from build123d import *
from OCP.BRepFilletAPI import BRepFilletAPI_MakeChamfer

# Parameters (mm, degrees)
SZKIC1_W                        = 58
SZKIC1_H                        = 20
DODANIE_WYCI_GNI_CIE1_DEPTH     = 5
SZKIC2_W                        = 15
SZKIC2_H                        = 5
DODANIE_WYCI_GNI_CIE2_DEPTH     = 58
DODANIE_WYCI_GNI_CIE3_DEPTH     = 20
DODANIE_WYCI_GNI_CIE4_DEPTH     = 10
WYTNIJ_WYCI_GNI_CIE2_DEPTH      = 50.950375374
WYTNIJ_WYCI_GNI_CIE2_DEPTH_BACK = 50.950375374
SZKIC6_W                        = 58
SZKIC6_H                        = 5
DODANIE_WYCI_GNI_CIE5_DEPTH     = 20
SZKIC7_R                        = 2
WYTNIJ_WYCI_GNI_CIE3_DEPTH      = 10
DODANIE_WYCI_GNI_CIE8_DEPTH     = 10
SZKIC11_W                       = 10.2
SZKIC11_H                       = 10.2
DODANIE_WYCI_GNI_CIE9_DEPTH     = 5
SFAZOWANIE2_SIZE                = 5
SZKIC12_W                       = 10
SZKIC12_H                       = 20
WYTNIJ_WYCI_GNI_CIE4_DEPTH      = 10
SZKIC13_R                       = 1.7
WYTNIJ_WYCI_GNI_CIE5_DEPTH      = 60.991999467
DODANIE_WYCI_GNI_CIE11_DEPTH    = 5
SFAZOWANIE6_SIZE                = 5
SFAZOWANIE6_SIZE2               = 8.660254038


with BuildPart() as part:
    # Szkic1 → Dodanie-wyciągnięcie1 (new body)
    with BuildSketch(Plane.XY):
        Rectangle(SZKIC1_W, SZKIC1_H)
    extrude(amount=DODANIE_WYCI_GNI_CIE1_DEPTH)

    # Szkic2 → Dodanie-wyciągnięcie2 (add)
    with BuildSketch(Plane(origin=(29, 0, 0), x_dir=(0, 0, -1), z_dir=(1, 0, 0))):
        with Locations((-2.5, 12.5)):
            Rectangle(SZKIC2_W, SZKIC2_H)
    extrude(amount=-DODANIE_WYCI_GNI_CIE2_DEPTH)

    # Szkic3 → Dodanie-wyciągnięcie3 (add)
    with BuildSketch(Plane.XZ.offset(10)):
        Polygon((-34, 5), (-29, 0), (-29, 5), (-24, 5), (-29, 10), (-34, 10), align=None)
    extrude(amount=-DODANIE_WYCI_GNI_CIE3_DEPTH)

    # Szkic5 → Dodanie-wyciągnięcie4 (add)
    with BuildSketch(Plane.XY.offset(5)):
        Polygon((14.2, 20.2), (14.2, 10), (19, 10), (19, 35.2), (-16, 35.2), (-16, 10), (4, 10), (4, 20.2), align=None)
    extrude(amount=-DODANIE_WYCI_GNI_CIE4_DEPTH)

    # Szkic5<3> → Wytnij-wyciągnięcie2 (cut, two sides: drawn at the far end of the back side and taken through both)
    with BuildSketch(Plane.XY.offset(5).offset(-WYTNIJ_WYCI_GNI_CIE2_DEPTH_BACK)):
        Polygon((4, 10), (14.2, 10), (14.2, 15), (14.2, 20.2), (4, 20.2), (4, 15), align=None)
    extrude(amount=WYTNIJ_WYCI_GNI_CIE2_DEPTH + WYTNIJ_WYCI_GNI_CIE2_DEPTH_BACK, mode=Mode.SUBTRACT)

    # Szkic6 → Dodanie-wyciągnięcie5 (add)
    with BuildSketch(Plane(origin=(0, 10, 0), x_dir=(1, 0, 0), z_dir=(0, 1, 0))):
        with Locations((0, -7.5)):
            Rectangle(SZKIC6_W, SZKIC6_H)
    extrude(amount=-DODANIE_WYCI_GNI_CIE5_DEPTH)

    # Szkic7 → Wytnij-wyciągnięcie3 (cut)
    with BuildSketch(Plane.XZ.offset(10)):
        with Locations(Location((-19, 5, 0), (0, 0, 270))):
            Circle(SZKIC7_R)
        with Locations(Location((11, 5, 0), (0, 0, 270))):
            Circle(SZKIC7_R)
    extrude(amount=-WYTNIJ_WYCI_GNI_CIE3_DEPTH, mode=Mode.SUBTRACT)

    # Szkic10 → Dodanie-wyciągnięcie8 (add)
    with BuildSketch(Plane(origin=(0, 0, -5), x_dir=(-1, 0, 0), z_dir=(0, 0, -1))):
        Polygon((16, 10), (16, 15), (16, 35.2), (-19, 35.2), (-19, 15), (-29, 15), (-29, 10), (-14.2, 10), (-14.2, 20.2), (-4, 20.2), (-4, 10), align=None)
    extrude(amount=DODANIE_WYCI_GNI_CIE8_DEPTH)

    # Szkic11 → Dodanie-wyciągnięcie9 (add)
    with BuildSketch(Plane(origin=(0, 0, -15), x_dir=(-1, 0, 0), z_dir=(0, 0, -1))):
        with Locations((-9.1, 15.1)):
            Rectangle(SZKIC11_W, SZKIC11_H)
        Polygon((-29, 10), (-14.2, 10), (-14.2, 20.2), (-4, 20.2), (-4, 10), (16, 10), (16, 35.2), (-19, 35.2), (-19, 15), (-29, 15), align=None)
    extrude(amount=DODANIE_WYCI_GNI_CIE9_DEPTH)

    # Sfazowanie2
    sfazowanie2_edges = [part.edges().sort_by_distance(p)[0] for p in [
        (-16, 35.2, -7.5),
        (19, 35.2, -7.5),
    ]]
    chamfer(sfazowanie2_edges, length=SFAZOWANIE2_SIZE)

    # Szkic12 → Wytnij-wyciągnięcie4 (cut)
    with BuildSketch(Plane.XZ.offset(-10)):
        with Locations((24, -10)):
            Rectangle(SZKIC12_W, SZKIC12_H)
    extrude(amount=-WYTNIJ_WYCI_GNI_CIE4_DEPTH, mode=Mode.SUBTRACT)

    # Szkic13 → Wytnij-wyciągnięcie5 (cut, through all)
    with BuildSketch(Plane(origin=(0, 35.2, 0), x_dir=(1, 0, 0), z_dir=(0, 1, 0))):
        with Locations(Location((9.1, 3, 0), (0, 0, 270))):
            Circle(SZKIC13_R)
    extrude(amount=-WYTNIJ_WYCI_GNI_CIE5_DEPTH, mode=Mode.SUBTRACT)

    # Szkic15 → Dodanie-wyciągnięcie11 (add)
    with BuildSketch(Plane.XY.offset(5)):
        Polygon((19, 15), (19, 30.2), (14, 35.2), (-11, 35.2), (-16, 30.2), (-16, 15), (4, 15), (4, 20.2), (14.2, 20.2), (14.2, 15), align=None)
    extrude(amount=DODANIE_WYCI_GNI_CIE11_DEPTH)

    # Sfazowanie6: one chamfer whose edges measure the first distance from different faces: ONE call of the kernel's chamfer builder (chamfer() names one face for all edges)
    sfazowanie6_edges_1 = [part.edges().sort_by_distance(p)[0] for p in [
        (-16, 15, 2.5),
    ]]
    sfazowanie6_side_1 = [part.faces().sort_by_distance(p)[0] for p in [
        (-22.5, 15, 2.5),
    ]]
    sfazowanie6_edges_2 = [part.edges().sort_by_distance(p)[0] for p in [
        (19, 15, 5),
    ]]
    sfazowanie6_side_2 = [part.faces().sort_by_distance(p)[0] for p in [
        (24, 15, 5),
    ]]
    sfazowanie6 = BRepFilletAPI_MakeChamfer(part.part.solid().wrapped)
    for e in sfazowanie6_edges_1:
        sfazowanie6.Add(SFAZOWANIE6_SIZE, SFAZOWANIE6_SIZE2, e.wrapped, sfazowanie6_side_1[0].wrapped)  # the first distance lies on this face
    for e in sfazowanie6_edges_2:
        sfazowanie6.Add(SFAZOWANIE6_SIZE, SFAZOWANIE6_SIZE2, e.wrapped, sfazowanie6_side_2[0].wrapped)  # the first distance lies on this face
    add(Compound.cast(sfazowanie6.Shape()), mode=Mode.REPLACE)


solid = part.part
The model under review builds one solid part; all positions refer to its coordinate system, in mm. A direction names the side the tool comes from. Give positions to 0.01 mm unless a question says otherwise; leave off trailing zeros. Write each loop counter-clockwise with the first axis right and the second up, starting at its lowest first coordinate (ties: lowest second). Pieces come first, ordered by that corner, then holes.
1. Add section D-D, the plane y = 11.5. Write out the cut boundary in (x, z).
2. Wall thickness on L1, parallel to X at y = -5, z = 5; L2, parallel to Y at x = 4.5, z = 6.5; L3, parallel to X at y = 28.5, z = -3: over which ranges is each line inside the solid? List them lowest first.
3. Add section B-B, the plane z = 6.25. Write out the cut boundary in (x, y).
4. For P1, Ø1.5, axis at y = 13.5, z = 1.5, coming from the -X side; P2, Ø6.5, axis at x = -25.5, z = 1, coming from the +Y side; P3, Ø8, axis at y = 14, z = -14, coming from the +X side; P4, Ø4.5, axis at x = 9.1, z = -3, coming from the +Y side, all flat-tipped, find the tip position at first contact; note any pin that passes through.
5. Draft analysis for pull direction Y (two halves, no side actions). For faces 6 (the flat face through (-5, 10, -10)), 7 (the flat face through (14.2, 15, -3)), 8 (the flat face through (26, 15, 5)), state which applies: +Y half, -Y half, draft (parallel to the pull), parting line (faces both ways), or undercut.
6. Tool access review of faces 1 (the flat face through (16.5, 32.7, -5.2)), 2 (the flat face through (-25, 15, 3)), 3 (the flat face through (9, 10, 5)), 4 (the flat face through (11, 0, 5)), 5 (the flat face through (-21, 14, -5)): name each direction out of +Z, -Z, +X, -X, +Y, -Y from which nothing blocks a thin tool from reaching the whole face with its end or side.
7. Add section C-C, the plane x = 12. Write out the cut boundary in (y, z), plus the area to 3 significant figures.
8. Add section A-A, the plane y = 25. Write out the cut boundary in (x, z), plus the area to 3 significant figures.
Worked answers:
1. outline: (-29, -5) - (-16, -5) - (-16, -20) - (19, -20) - (19, 0) - (29, 0) - (29, 10) - (14.2, 10) - (14.2, -15) - (4, -15) - (4, 10) - (-29, 10) - close
2. L1: x = -34 to -21, -17 to 9, 13 to 29
2. L2: y = -10 to 10, 20.2 to 35.2
2. L3: x = -16 to 7.4, 10.8 to 19
3. outline: (-34, -10) - (-20.56, -10) - (-20.56, 0) - (-17.44, 0) - (-17.44, -10) - (9.44, -10) - (9.44, 0) - (12.56, 0) - (12.56, -10) - (29, -10) - (29, 15) - (24, 15) - (19, 23.66) - (19, 30.2) - (14, 35.2) - (-11, 35.2) - (-16, 30.2) - (-16, 23.66) - (-21, 15) - (-29, 15) - (-29, 10) - (-34, 10) - close; hole (4, 10) - (14.2, 10) - (14.2, 20.2) - (4, 20.2) - close
4. P1: stops at x = -29
4. P2: stops at y = 15
4. P3: stops at x = 19
4. P4: stops at y = 35.2
5. face 6: -Y half
5. face 7: undercut
5. face 8: +Y half
6. face 1: +Z, -Z, +X, +Y
6. face 2: +Z, -Z, -X, +Y
6. face 3: +Z
6. face 4: -Y
6. face 5: -Z, -X, +Y, -Y
7. outline: (-10, 0) - (10, 0) - (10, 10) - (-10, 10) - (-10, 6.73) - (0, 6.73) - (0, 3.27) - (-10, 3.27) - close; (10, -20) - (35.2, -20) - (35.2, 10) - (20.2, 10) - (20.2, -15) - (10, -15) - close
7. area: 666 mm2
8. outline: (-16, -20) - (19, -20) - (19, 10) - (-16, 10) - close; hole circle Ø3.4 at (9.1, -3)
8. area: 1,040 mm2
